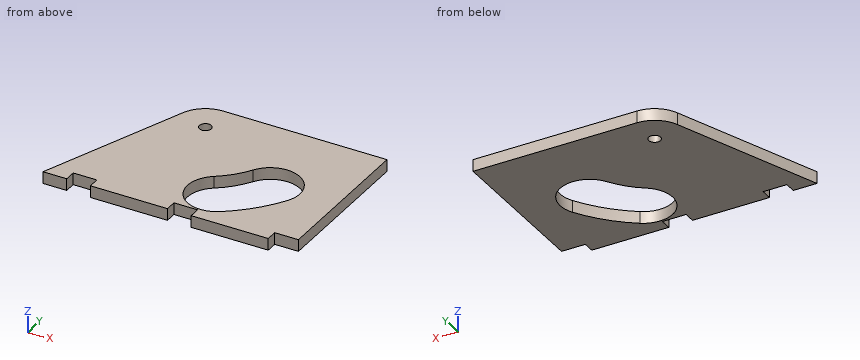
```python
from build123d import *

# Parameters (mm, degrees)
SKETCH1_W           = 120
SKETCH1_H           = 100
BOSS_EXTRUDE1_DEPTH = 5
SKETCH2_R           = 2.5
CUT_EXTRUDE1_DEPTH  = 6
SKETCH3_W           = 120
SKETCH3_H           = 2
BOSS_EXTRUDE2_DEPTH = 20
CUT_EXTRUDE2_DEPTH  = 26
CUT_EXTRUDE3_DEPTH  = 26
SKETCH6_W           = 5
SKETCH6_H           = 30
BOSS_EXTRUDE3_DEPTH = 20
CUT_EXTRUDE4_DEPTH  = 106
SKETCH10_W          = 27.884556649
SKETCH10_H          = 70
CUT_EXTRUDE5_DEPTH  = 106
SKETCH11_W          = 20
SKETCH11_H          = 30
CUT_EXTRUDE6_DEPTH  = 106
SKETCH12_W          = 10
SKETCH12_H          = 4.75
CUT_EXTRUDE7_DEPTH  = 6


with BuildPart() as part:
    # Sketch1 → Boss-Extrude1 (new body)
    with BuildSketch(Plane.XY):
        with Locations((60, 50)):
            Rectangle(SKETCH1_W, SKETCH1_H)
    boss_extrude1 = extrude(amount=BOSS_EXTRUDE1_DEPTH)

    # Sketch2 → Cut-Extrude1 (cut, through all)
    with BuildSketch(Plane.XY.offset(5)):
        with Locations((50.878001036, 56.909722104)):
            Circle(SKETCH2_R)
        with BuildLine():
            ThreePointArc((85.292587217, 7.760599446), (95.03577446, 16.288409394), (102.722518982, 26.707967867))
            ThreePointArc((102.722518982, 26.707967867), (98.213609876, 43.800941239), (81.120636505, 39.292032133))
            ThreePointArc((81.120636505, 39.292032133), (76.6367022, 33.213956356), (70.953176308, 28.239400554))
            ThreePointArc((70.953176308, 28.239400554), (67.883481209, 10.830294546), (85.292587217, 7.760599446))
        make_face()
    cut_extrude1 = extrude(amount=-CUT_EXTRUDE1_DEPTH, mode=Mode.SUBTRACT)

    # Sketch3 → Boss-Extrude2 (add)
    with BuildSketch(Plane(origin=(0, 0, 0), x_dir=(-1, 0, 0), z_dir=(0, 0, -1))):
        with Locations((-60, 1)):
            Rectangle(SKETCH3_W, SKETCH3_H)
    boss_extrude2 = extrude(amount=BOSS_EXTRUDE2_DEPTH)

    # Sketch4 → Cut-Extrude2 (cut, through all)
    with BuildSketch(Plane.XY.offset(5)):
        with BuildLine():
            ThreePointArc((71.705399269, 35.987211382), (76.514173113, 43.433069144), (75.177144341, 52.195343835))
            ThreePointArc((75.177144341, 52.195343835), (71.771162127, 53.143650303), (70.822855659, 49.737668089))
            ThreePointArc((70.822855659, 49.737668089), (71.625072922, 44.480303275), (68.739808616, 40.012788618))
            ThreePointArc((68.739808616, 40.012788618), (68.209815325, 36.517204673), (71.705399269, 35.987211382))
        make_face()
    extrude(amount=-CUT_EXTRUDE2_DEPTH, mode=Mode.SUBTRACT)

    # Sketch5 → Cut-Extrude3 (cut, through all)
    with BuildSketch(Plane.XY.offset(5)):
        with BuildLine():
            Line((120, 70), (50.878001036, 70))
            ThreePointArc((50.878001036, 70), (43.464411706, 67.698330385), (38.657892056, 61.602728806))
            Line((38.657892056, 61.602728806), (15, 0))
            Line((15, 0), (0, 0))
            Line((0, 0), (0, 100))
            Line((0, 100), (120, 100))
            Line((120, 100), (120, 70))
        make_face()
    cut_extrude3 = extrude(amount=-CUT_EXTRUDE3_DEPTH, mode=Mode.SUBTRACT)

    # Sketch6 → Boss-Extrude3 (add, through all)
    with BuildSketch(Plane(origin=(0, 0, 0), x_dir=(-1, 0, 0), z_dir=(0, 0, -1))):
        with Locations((-117.5, 15)):
            Rectangle(SKETCH6_W, SKETCH6_H)
        with Locations((-32.5, 15)):
            Rectangle(SKETCH6_W, SKETCH6_H)
    boss_extrude3 = extrude(amount=BOSS_EXTRUDE3_DEPTH)

    # Sketch9 → Cut-Extrude4 (cut, through all)
    with BuildSketch(Plane(origin=(120, 0, 0), x_dir=(0, 0, -1), z_dir=(1, 0, 0))):
        Polygon((0, 30), (20, 0), (20, 30), align=None)
    cut_extrude4 = extrude(amount=-CUT_EXTRUDE4_DEPTH, mode=Mode.SUBTRACT)

    # Mirror1: Boss-Extrude1, Cut-Extrude1, Boss-Extrude2, Cut-Extrude3, Boss-Extrude3, Cut-Extrude4 across plane
    add(boss_extrude1.mirror(Plane(origin=(0, 0, 5), x_dir=(1, 0, 0), z_dir=(0, 0, -1))))
    add(cut_extrude1.mirror(Plane(origin=(0, 0, 5), x_dir=(1, 0, 0), z_dir=(0, 0, -1))), mode=Mode.SUBTRACT)
    add(boss_extrude2.mirror(Plane(origin=(0, 0, 5), x_dir=(1, 0, 0), z_dir=(0, 0, -1))))
    add(cut_extrude3.mirror(Plane(origin=(0, 0, 5), x_dir=(1, 0, 0), z_dir=(0, 0, -1))), mode=Mode.SUBTRACT)
    add(boss_extrude3.mirror(Plane(origin=(0, 0, 5), x_dir=(1, 0, 0), z_dir=(0, 0, -1))))
    add(cut_extrude4.mirror(Plane(origin=(0, 0, 5), x_dir=(1, 0, 0), z_dir=(0, 0, -1))), mode=Mode.SUBTRACT)

    # Sketch10 → Cut-Extrude5 (cut, through all)
    with BuildSketch(Plane(origin=(120, 0, 0), x_dir=(0, 0, -1), z_dir=(1, 0, 0))):
        with Locations((8.942278325, 35)):
            Rectangle(SKETCH10_W, SKETCH10_H)
    extrude(amount=-CUT_EXTRUDE5_DEPTH, mode=Mode.SUBTRACT)

    # Sketch11 → Cut-Extrude6 (cut, through all)
    with BuildSketch(Plane(origin=(120, 0, 0), x_dir=(0, 0, -1), z_dir=(1, 0, 0))):
        with Locations((-20, 15)):
            Rectangle(SKETCH11_W, SKETCH11_H)
    extrude(amount=-CUT_EXTRUDE6_DEPTH, mode=Mode.SUBTRACT)

    # Sketch12 → Cut-Extrude7 (cut, through all)
    with BuildSketch(Plane.XY.offset(10)):
        with Locations((115, 2.375)):
            Rectangle(SKETCH12_W, SKETCH12_H)
        with Locations((72.5, 2.375)):
            Rectangle(SKETCH12_W, SKETCH12_H)
        with Locations((30, 2.375)):
            Rectangle(SKETCH12_W, SKETCH12_H)
    extrude(amount=-CUT_EXTRUDE7_DEPTH, mode=Mode.SUBTRACT)


solid = part.part
```
Build history of the part. All positions in model axes, mm. Round coordinates to 2 decimals unless told otherwise and drop trailing zeros. Write each loop counter-clockwise with the first axis right and the second up, starting at its lowest first coordinate (ties: lowest second). Pieces come first, ordered by that corner, then holes.
1) Drill centre lines: probe 1 along X at (y, z) = (18, 5.7); probe 2 along X at (y, z) = (23, 5.9); probe 3 along Y at (x, z) = (50, 7.05). Where is each one in solid material? Low to high.
2) Band-saw the part on B-B, the plane y = 36. List the corners of the cut face in (x, z), and give its area (3 significant figures).
3) Band-saw the part on C-C, the plane z = 6.9. List the corners of the cut face in (x, y), and give its area (3 significant figures).
4) Band-saw the part on A-A, the plane x = 83.5. List the corners of the cut face in (y, z).
5) Pin check, flat tips, straight feed: pin 1 (2.5 mm diameter, centred on x = 29.5, z = 6.5, fed in from -Y); pin 2 (2.5 mm diameter, centred on y = 3.5, z = 8, fed in from -X). Stop position of each tip, or through.
6) Band-saw the part on D-D, the plane x = 33. List the corners of the cut face in (y, z), and give its area (3 significant figures).
Ans:
1. probe 1: x = 21.91 to 65.62, 96.55 to 120
1. probe 2: x = 23.83 to 66.67, 100.38 to 120
1. probe 3: y = 0 to 54.57, 59.25 to 69.97
2. outline: (28.83, 5) - (78.95, 5) - (78.95, 10) - (28.83, 10) - close; (104.06, 5) - (120, 5) - (120, 10) - (104.06, 10) - close
2. area: 330 mm2
3. outline: (15, 0) - (25, 0) - (25, 4.75) - (35, 4.75) - (35, 0) - (67.5, 0) - (67.5, 4.75) - (77.5, 4.75) - (77.5, 0) - (110, 0) - (110, 4.75) - (120, 4.75) - (120, 70) - (50.88, 70) arc R13.09 ccw to (38.66, 61.6) - close; hole circle Ø5 at (50.88, 56.91); hole (70.95, 28.24) arc R12.5 ccw to (85.29, 7.76) arc R60 ccw to (102.72, 26.71) arc R12.5 ccw to (81.12, 39.29) arc R35 cw to start
3. area: 5,230 mm2
4. outline: (0, 5) - (6.72, 5) - (6.72, 10) - (0, 10) - close; (42.24, 5) - (70, 5) - (70, 10) - (42.24, 10) - close
5. pin 1: stops at y = 4.75
5. pin 2: stops at x = 15.86
6. outline: (4.75, 5) - (46.87, 5) - (46.87, 10) - (4.75, 10) - close
6. area: 211 mm2
